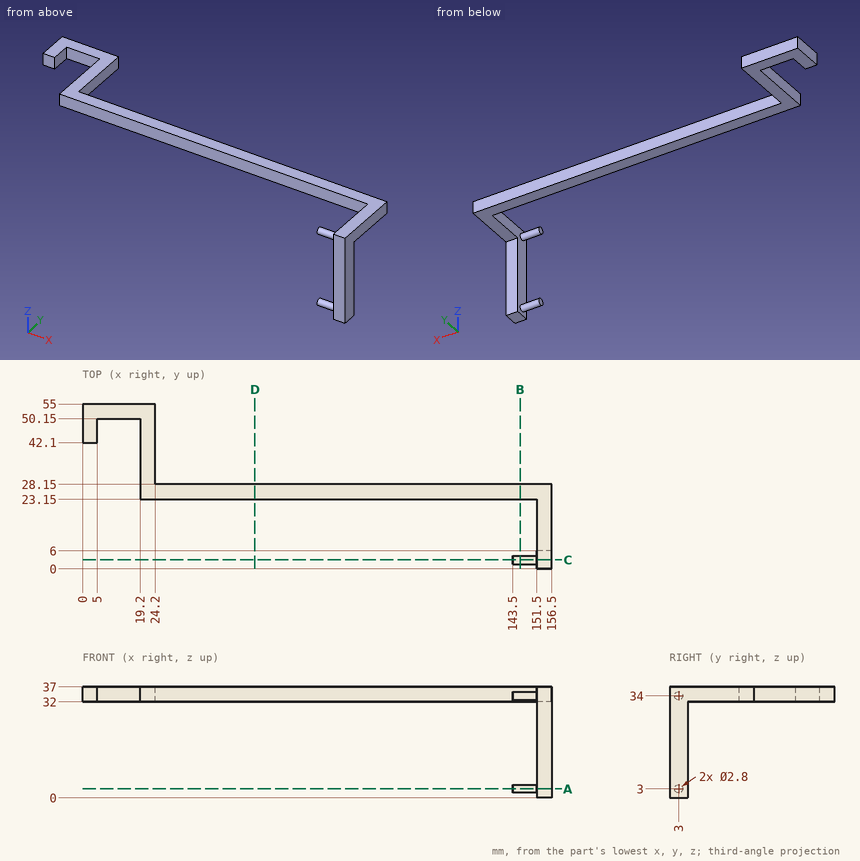
Here's the drawing with two shaded views (mm, measured from the low corner). I have some questions. Coordinates: 2 decimals unless noted, no trailing zeros. Order: outer loops, then holes, each group sorted by start corner. A loop starts at its lowest first (then second) coordinate and runs counter-clockwise, first axis right, second up. Notation, with made-up numbers: M 15.5,41.25 L 72.5,41.25 A23 cw 72.5,57.25 Z; hole C -4.5,-1 d2. An arc over 180 degrees is marked long. Write item = value, one per line.
(1) Suppose I cut it at D-D on x = 57.5. Please give me the cut outline in (y, z), plus the area to 3 significant figures.
Results are:
outline = M 23.15,32 L 28.15,32 L 28.15,37 L 23.15,37 Z
area = 25.0 mm2
(2) For pin 1 Ø2 at (y, z) = (3, 34.5) entering from -X; pin 2 Ø8 at (x, y) = (105.5, 20) entering from +Z; pin 3 Ø2.5 at (y, z) = (35.5, 33.5) entering from -X; pin 4 Ø12 at (x, y) = (74.5, 13.5) entering from -Z, each with a flat end and sliding along its axis, tell me the tip position at first contact or that it passes through.
Results are:
pin_1 = 143.5
pin_2 = 37
pin_3 = 19.2
pin_4 = through
(3) Suppose I cut it at C-C on y = 3. Please give me the cut outline in (x, z), plus the area to 3 significant figures.
Results are:
outline = M 143.5,1.6 L 151.5,1.6 L 151.5,0 L 156.5,0 L 156.5,37 L 151.5,37 L 151.5,35.4 L 143.5,35.4 L 143.5,32.6 L 151.5,32.6 L 151.5,4.4 L 143.5,4.4 Z
area = 230 mm2
(4) Suppose I cut it at A-A on z = 3. Please give me the cut outline in (x, y).
Results are:
outline = M 143.5,1.6 L 151.5,1.6 L 151.5,0 L 156.5,0 L 156.5,6 L 151.5,6 L 151.5,4.4 L 143.5,4.4 Z
(5) I need wall thicknesses on line 1 along Z through (x, y) = (56, 27); line 2 along Y through (x, z) = (82, 34.5); line 3 along X through (y, z) = (5.5, 30.5). Which ranges of each line are inside material? Lowest first, please. Write a range as [from, to].
Results are:
line_1 = [32, 37]
line_2 = [23.15, 28.15]
line_3 = [151.5, 156.5]
(6) Suppose I cut it at B-B on x = 146. Please give me the cut outline in (y, z), plus the area to 3 significant figures.
Results are:
outline = C 3,3 d2.8; C 3,34 d2.8; M 23.15,32 L 28.15,32 L 28.15,37 L 23.15,37 Z
area = 37.3 mm2
